Here's how the part is built. I have some questions about the finished solid (model axes, mm). A direction names the side the tool comes from. Round coordinates to 2 decimals unless told otherwise and drop trailing zeros. Order: outer loops, then holes, each group sorted by start corner. A loop starts at its lowest first (then second) coordinate and runs counter-clockwise, first axis right, second up. Notation, with made-up numbers: (40.25, 33) - (47.25, 33) arc R18 ccw to (47.25, 46) - close; hole circle Ø3 at (89, 16). An arc over 180 degrees is marked (long way). Answer as a JSON object with one key per item and string values.
```python
from build123d import *

# Parameters (mm, degrees)
SKETCH002_W          = 150
SKETCH002_H          = 150
PAD002_DEPTH         = 6
POCKET_DEPTH         = 0.001
POCKET_DEPTH_BACK    = 6.001
SKETCH004_R          = 2.5
POCKET001_DEPTH      = 6.001
POCKET001_DEPTH_BACK = 0.001


with BuildPart() as part:
    # Sketch002 → Pad002 (new body)
    with BuildSketch(Plane.XY):
        Rectangle(SKETCH002_W, SKETCH002_H)
    extrude(amount=PAD002_DEPTH)

    # Sketch003 → Pocket (cut, two sides)
    with BuildSketch(Plane.XY) as pocket_sk:
        Polygon((-60, 40), (-40, 60), (40, 60), (60, 40), (60, -40), (40, -60), (-40, -60), (-60, -40), align=None)
    extrude(amount=-POCKET_DEPTH, mode=Mode.SUBTRACT)
    extrude(pocket_sk.sketch, amount=POCKET_DEPTH_BACK, mode=Mode.SUBTRACT)

    # Sketch004 (on Face5 of Pad002) → Pocket001 (cut, two sides)
    with BuildSketch(Plane(origin=(0, 0, 0), x_dir=(1, 0, 0), z_dir=(0, 0, -1))) as pocket001_sk:
        with Locations((-63, 63)):
            Circle(SKETCH004_R)
        with Locations((63, 63)):
            Circle(SKETCH004_R)
        with Locations((63, -63)):
            Circle(SKETCH004_R)
        with Locations((-63, -63)):
            Circle(SKETCH004_R)
    extrude(amount=-POCKET001_DEPTH, mode=Mode.SUBTRACT)
    extrude(pocket001_sk.sketch, amount=POCKET001_DEPTH_BACK, mode=Mode.SUBTRACT)


solid = part.part
```
1. Imagine slicing it at B-B (y = -52). List the corners of the cut face in (x, z) for me.
Responses:
{"outline": "(-75, 0) - (-48, 0) - (-48, 6) - (-75, 6) - close; (48, 0) - (75, 0) - (75, 6) - (48, 6) - close"}
2. Imagine slicing it at D-D (x = 63). List the corners of the cut face in (y, z) for me, plus the area to 3 significant figures.
Responses:
{"outline": "(-75, 0) - (-65.5, 0) - (-65.5, 6) - (-75, 6) - close; (-60.5, 0) - (60.5, 0) - (60.5, 6) - (-60.5, 6) - close; (65.5, 0) - (75, 0) - (75, 6) - (65.5, 6) - close", "area": "840 mm2"}
3. Thinking about a two-plate mould opening in X: for faces 3 (the face through (-1, -75, 3)), 4 (the face through (-75, -1, 3)), 5 (the face through (-60.69, -62.04, 2.96)), 6 (the face through (75, -1, 3)), which applies, pulls with the +X half, pulls with the -X half, needs draft (parallel to the pull), parting line crosses it, or undercut?
Responses:
{"face 3": "needs draft", "face 4": "pulls with the -X half", "face 5": "undercut", "face 6": "pulls with the +X half"}
4. Imagine slicing it at C-C (z = 1.25). List the corners of the cut face in (x, y) for me, plus the area to 3 significant figures.
Responses:
{"outline": "(-75, -75) - (75, -75) - (75, 75) - (-75, 75) - close; hole circle Ø5 at (-63, -63); hole circle Ø5 at (-63, 63); hole (-60, -40) - (-40, -60) - (40, -60) - (60, -40) - (60, 40) - (40, 60) - (-40, 60) - (-60, 40) - close; hole circle Ø5 at (63, -63); hole circle Ø5 at (63, 63)", "area": "8,820 mm2"}
5. Imagine slicing it at A-A (x = -51). List the corners of the cut face in (y, z) for me.
Responses:
{"outline": "(-75, 0) - (-49, 0) - (-49, 6) - (-75, 6) - close; (49, 0) - (75, 0) - (75, 6) - (49, 6) - close"}
6. For faces 1 (the face through (-1, 75, 3)), 2 (the face through (50, 50, 3)), which set-ups out of +Z, -Z, +X, -X, +Y, -Y let a thin tool reach every point of the face, with its end or its side?
Responses:
{"face 1": "+Z, -Z, +X, -X, +Y", "face 2": "+Z, -Z"}
7. If I drill on L1, parallel to X at y = 63, z = 3.6; L2, parallel to X at y = -61.5, z = 1.75, over which ranges is the centre line in solid material (lowest first)? Write a range as [from, to].
Responses:
{"L1": "[-75, -65.5], [-60.5, 60.5], [65.5, 75]", "L2": "[-75, -65], [-61, 61], [65, 75]"}
